Work out the finished part from the listing and answer in its coordinate system (mm). A direction names the side the tool comes from. Round coordinates to 2 decimals unless told otherwise and drop trailing zeros. Loops run counter-clockwise (first coordinate to the right, second up) from the corner with the lowest first, then second, coordinate; pieces in that order, holes last. Notation, with made-up numbers: (50, 39) - (103, 39) arc R15 cw to (103, 68) - close; hole circle Ø3 at (70.25, -35). An arc over 180 degrees is marked (long way). Return JSON: item names as keys, results as strings.
from build123d import *
from OCP.BRepFilletAPI import BRepFilletAPI_MakeChamfer

# Parameters (mm, degrees)
SKETCH1_W           = 28
SKETCH1_H           = 27
BOSS_EXTRUDE1_DEPTH = 2
SKETCH2_W           = 10
SKETCH2_H           = 2.5
CUT_EXTRUDE1_DEPTH  = 2
SKETCH3_W           = 20
SKETCH3_H           = 14.5
BOSS_EXTRUDE2_DEPTH = 3
SKETCH4_W           = 24
SKETCH4_H           = 23
SKETCH4_W_2         = 20
SKETCH4_H_2         = 19
BOSS_EXTRUDE3_DEPTH = 6
SKETCH5_R           = 0.95
CUT_EXTRUDE2_DEPTH  = 3.2
FILLET3_R           = 2
FILLET2_R           = 0.5
SKETCH6_W           = 27
SKETCH6_H           = 2
BOSS_EXTRUDE4_DEPTH = 70
CHAMFER1_SIZE       = 3.5
CHAMFER1_SIZE2      = 0.306210322
SKETCH7_W           = 28
SKETCH7_H           = 2.1
CUT_EXTRUDE3_DEPTH  = 86.289213855
SKETCH8_W           = 40
SKETCH8_H           = 8
BOSS_EXTRUDE5_DEPTH = 2


with BuildPart() as part:
    # Sketch1 → Boss-Extrude1 (new body)
    with BuildSketch(Plane(origin=(0, 0, 0), x_dir=(1, 0, 0), z_dir=(0, 1, 0))):
        Rectangle(SKETCH1_W, SKETCH1_H)
    extrude(amount=BOSS_EXTRUDE1_DEPTH)

    # Sketch2 → Cut-Extrude1 (cut)
    with BuildSketch(Plane(origin=(0, 2, 0), x_dir=(1, 0, 0), z_dir=(0, 1, 0))):
        with Locations((3, 7.25)):
            Rectangle(SKETCH2_W, SKETCH2_H)
    extrude(amount=-CUT_EXTRUDE1_DEPTH, mode=Mode.SUBTRACT)

    # Sketch3 → Boss-Extrude2 (add)
    with BuildSketch(Plane(origin=(0, 2, 0), x_dir=(1, 0, 0), z_dir=(0, 1, 0))):
        with Locations((0, -2.25)):
            Rectangle(SKETCH3_W, SKETCH3_H)
    extrude(amount=BOSS_EXTRUDE2_DEPTH)

    # Sketch4 → Boss-Extrude3 (add)
    with BuildSketch(Plane(origin=(0, 2, 0), x_dir=(1, 0, 0), z_dir=(0, 1, 0))):
        Rectangle(SKETCH4_W, SKETCH4_H)
        Rectangle(SKETCH4_W_2, SKETCH4_H_2, mode=Mode.SUBTRACT)
    extrude(amount=BOSS_EXTRUDE3_DEPTH)

    # Sketch5 → Cut-Extrude2 (cut)
    with BuildSketch(Plane(origin=(0, 5, 0), x_dir=(1, 0, 0), z_dir=(0, 1, 0))):
        with Locations(Location((-7, -6.5, 0), (0, 0, 270))):
            Circle(SKETCH5_R)
        with Locations(Location((7, -6.5, 0), (0, 0, 90))):
            Circle(SKETCH5_R)
    extrude(amount=-CUT_EXTRUDE2_DEPTH, mode=Mode.SUBTRACT)

    # Fillet3
    fillet3_edges = [part.edges().sort_by_distance(p)[0] for p in [
        (12, 5, -11.5),
        (-12, 5, -11.5),
        (-12, 5, 11.5),
        (12, 5, 11.5),
        (14, 1, 13.5),
        (14, 1, -13.5),
    ]]
    fillet(fillet3_edges, radius=FILLET3_R)

    # Fillet2
    fillet2_edges = [part.edges().sort_by_distance(p)[0] for p in [
        (-2, 1, -8.5),
        (-2, 1, -6),
        (8, 1, -6),
        (8, 1, -8.5),
        (10, 5, -9.5),
        (-10, 6.5, 9.5),
        (10, 6.5, 9.5),
        (-10, 5, -9.5),
    ]]
    fillet(fillet2_edges, radius=FILLET2_R)

    # Sketch6 → Boss-Extrude4 (add)
    with BuildSketch(Plane.ZY.offset(14)):
        with Locations((0, 1)):
            Rectangle(SKETCH6_W, SKETCH6_H)
    extrude(amount=BOSS_EXTRUDE4_DEPTH)

    # Chamfer1: one chamfer whose edges measure the first distance from different faces: ONE call of the kernel's chamfer builder (chamfer() names one face for all edges)
    chamfer1_edges_1 = [part.edges().sort_by_distance(p)[0] for p in [
        (0, 8, -11.5),
    ]]
    chamfer1_side_1 = [part.faces().sort_by_distance(p)[0] for p in [
        (0, 5, -11.5),
    ]]
    chamfer1_edges_2 = [part.edges().sort_by_distance(p)[0] for p in [
        (12, 8, 0),
    ]]
    chamfer1_side_2 = [part.faces().sort_by_distance(p)[0] for p in [
        (12, 5, 0),
    ]]
    chamfer1_edges_3 = [part.edges().sort_by_distance(p)[0] for p in [
        (-12, 8, 0),
    ]]
    chamfer1_side_3 = [part.faces().sort_by_distance(p)[0] for p in [
        (-12, 5, 0),
    ]]
    chamfer1_edges_4 = [part.edges().sort_by_distance(p)[0] for p in [
        (0, 8, 11.5),
    ]]
    chamfer1_side_4 = [part.faces().sort_by_distance(p)[0] for p in [
        (0, 5, 11.5),
    ]]
    chamfer1_edges_5 = [part.edges().sort_by_distance(p)[0] for p in [
        (-11.414213562, 8, -10.914213562),
    ]]
    chamfer1_side_5 = [part.faces().sort_by_distance(p)[0] for p in [
        (-11.414213562, 5, -10.914213562),
    ]]
    chamfer1_edges_6 = [part.edges().sort_by_distance(p)[0] for p in [
        (-11.414213562, 8, 10.914213562),
    ]]
    chamfer1_side_6 = [part.faces().sort_by_distance(p)[0] for p in [
        (-11.414213562, 5, 10.914213562),
    ]]
    chamfer1_edges_7 = [part.edges().sort_by_distance(p)[0] for p in [
        (11.414213562, 8, 10.914213562),
    ]]
    chamfer1_side_7 = [part.faces().sort_by_distance(p)[0] for p in [
        (11.414213562, 5, 10.914213562),
    ]]
    chamfer1_edges_8 = [part.edges().sort_by_distance(p)[0] for p in [
        (11.414213562, 8, -10.914213562),
    ]]
    chamfer1_side_8 = [part.faces().sort_by_distance(p)[0] for p in [
        (11.414213562, 5, -10.914213562),
    ]]
    chamfer1 = BRepFilletAPI_MakeChamfer(part.part.solid().wrapped)
    for e in chamfer1_edges_1:
        chamfer1.Add(CHAMFER1_SIZE, CHAMFER1_SIZE2, e.wrapped, chamfer1_side_1[0].wrapped)  # the first distance lies on this face
    for e in chamfer1_edges_2:
        chamfer1.Add(CHAMFER1_SIZE, CHAMFER1_SIZE2, e.wrapped, chamfer1_side_2[0].wrapped)  # the first distance lies on this face
    for e in chamfer1_edges_3:
        chamfer1.Add(CHAMFER1_SIZE, CHAMFER1_SIZE2, e.wrapped, chamfer1_side_3[0].wrapped)  # the first distance lies on this face
    for e in chamfer1_edges_4:
        chamfer1.Add(CHAMFER1_SIZE, CHAMFER1_SIZE2, e.wrapped, chamfer1_side_4[0].wrapped)  # the first distance lies on this face
    for e in chamfer1_edges_5:
        chamfer1.Add(CHAMFER1_SIZE, CHAMFER1_SIZE2, e.wrapped, chamfer1_side_5[0].wrapped)  # the first distance lies on this face
    for e in chamfer1_edges_6:
        chamfer1.Add(CHAMFER1_SIZE, CHAMFER1_SIZE2, e.wrapped, chamfer1_side_6[0].wrapped)  # the first distance lies on this face
    for e in chamfer1_edges_7:
        chamfer1.Add(CHAMFER1_SIZE, CHAMFER1_SIZE2, e.wrapped, chamfer1_side_7[0].wrapped)  # the first distance lies on this face
    for e in chamfer1_edges_8:
        chamfer1.Add(CHAMFER1_SIZE, CHAMFER1_SIZE2, e.wrapped, chamfer1_side_8[0].wrapped)  # the first distance lies on this face
    add(Compound.cast(chamfer1.Shape()), mode=Mode.REPLACE)

    # Sketch7 → Cut-Extrude3 (cut, through all)
    with BuildSketch(Plane(origin=(0, 2, 0), x_dir=(1, 0, 0), z_dir=(0, 1, 0))):
        with Locations((-70, 12.45)):
            Rectangle(SKETCH7_W, SKETCH7_H)
    cut_extrude3 = extrude(amount=-CUT_EXTRUDE3_DEPTH, mode=Mode.SUBTRACT)

    # Mirror1: Cut-Extrude3 across plane
    add(cut_extrude3.mirror(Plane.XY), mode=Mode.SUBTRACT)

    # Sketch8 → Boss-Extrude5 (add)
    with BuildSketch(Plane.XY.offset(13.5)):
        with Locations((-36, 6)):
            Rectangle(SKETCH8_W, SKETCH8_H)
    extrude(amount=-BOSS_EXTRUDE5_DEPTH)


solid = part.part
1) Section D-D (y = 9) is taken. Give the vertices of the cut face in (x, z).
Verdict:
{"outline": "(-56, 11.5) - (-16, 11.5) - (-16, 13.5) - (-56, 13.5) - close"}
2) Section B-B (z = 6.5) is taken. Give the vertices of the cut face in (x, y), and give its area (3 significant figures).
Verdict:
{"outline": "(-84, 0) - (14, 0) - (14, 2) - (12, 2) - (12, 4.5) - (11.69, 8) - (10, 8) - (10, 5) - (7.95, 5) - (7.95, 1.8) - (6.05, 1.8) - (6.05, 5) - (-6.05, 5) - (-6.05, 1.8) - (-7.95, 1.8) - (-7.95, 5) - (-10, 5) - (-10, 8) - (-11.69, 8) - (-12, 4.5) - (-12, 2) - (-84, 2) - close", "area": "267 mm2"}
3) Section C-C (x = -29) is taken. Give the vertices of the cut face in (y, z).
Verdict:
{"outline": "(0, -13.5) - (2, -13.5) - (2, 11.5) - (10, 11.5) - (10, 13.5) - (0, 13.5) - close"}
4) Section A-A (y = 3.5) is taken. Give the vertices of the cut face in (x, z).
Verdict:
{"outline": "(-56, 11.5) - (-16, 11.5) - (-16, 13.5) - (-56, 13.5) - close; (-12, -9.5) arc R2 ccw to (-10, -11.5) - (10, -11.5) arc R2 ccw to (12, -9.5) - (12, 9.5) arc R2 ccw to (10, 11.5) - (-10, 11.5) arc R2 ccw to (-12, 9.5) - close; hole (-10, -9) arc R0.5 ccw to (-9.5, -9.5) - (9.5, -9.5) arc R0.5 ccw to (10, -9) - (10, -5) - (-10, -5) - close; hole circle Ø1.9 at (-7, 6.5); hole circle Ø1.9 at (7, 6.5)"}
5) A tool of negligible diameter and unlimited length cuts with its end or side. For faces 1 (the flat face through (0, 3, 11.5)), 2 (the flat face through (-56, 5, 12)), 3 (the flat face through (0, 5, 2)), from which of +Z, -Z, +X, -X, +Y, -Y can it reach the whole face along a straight path? Write none if from no direction.
Verdict:
{"face 1": "+Z, +X, +Y", "face 2": "+Z, -X, +Y, -Y", "face 3": "+Y"}
6) Determine the mould class of faces 4 (the flat face through (-12, 3, 0)), 5 (the flat face through (-36, 6, 11.5)), 6 (the flat face through (7, 1.8, 7)) for opening direction Z: pulls with the +Z half, pulls with the -Z half, needs draft (parallel to the pull), parting line crosses it, or undercut.
Verdict:
{"face 4": "needs draft", "face 5": "pulls with the -Z half", "face 6": "undercut"}
7) Flat-ended cylindrical pins translate along their axes: pin 1 (2 mm diameter, centred on y = 1, z = -12.5, fed in from -X); pin 2 (3 mm diameter, centred on y = 6.5, z = -2, fed in from -X); pin 3 (2.5 mm diameter, centred on x = -0.5, y = 4, fed in from -Z); pin 4 (3 mm diameter, centred on y = 3, z = -7.5, fed in from -X). Find the tip coordinate at first contact, or state that the pin passes through.
Verdict:
{"pin 1": "stops at x = -56", "pin 2": "stops at x = -11.96", "pin 3": "stops at z = -11.5", "pin 4": "stops at x = -84"}
8) Find the intervals of material crossed by L1, parallel to X at y = 4.3, z = 6.5; L2, parallel to Z at x = 7, y = 3.35; L3, parallel to Y at x = -62, z = 2.5, in increasing order.
Verdict:
{"L1": "x = -12 to -7.95, -6.05 to 6.05, 7.95 to 12", "L2": "z = -11.5 to -9.5, -5 to 5.55, 7.45 to 11.5", "L3": "y = 0 to 2"}
